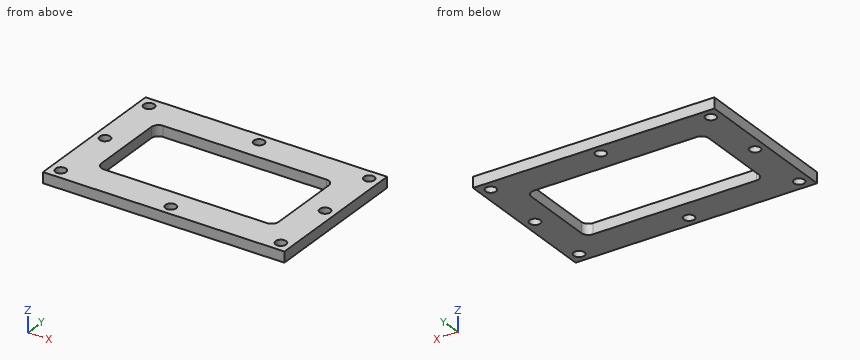
Autodesk Inventor part; units mm, degrees
ref_plane "YZ Plane" through (0, 0, 0) normal (1, 0, 0) x (0, 1, 0)
ref_plane "XZ Plane" through (0, 0, 0) normal (0, 1, 0) x (-1, 0, 0)
ref_plane "XY Plane" through (0, 0, 0) normal (0, 0, 1) x (1, 0, 0)
sketch "Sketch2" plane through (0, 0, 0) normal (0, 0, 1) x (1, 0, 0)
  line L0 (34, -21.5) -> (-34, -21.5)
  line L1 (-34, -21.5) -> (-34, 21.5)
  line L2 (-34, 21.5) -> (34, 21.5)
  line L3 (34, 21.5) -> (34, -21.5)
  line L4 (34, -21.5) -> (-34, 21.5) construction
  line L5 (-34, -21.5) -> (34, 21.5) construction
  line L6 (23, -12.5) -> (-23, -12.5)
  line L7 (-25, -10.5) -> (-25, 10.5)
  line L8 (-23, 12.5) -> (23, 12.5)
  line L9 (25, 10.5) -> (25, -10.5)
  line L10 (25, -12.5) -> (-25, 12.5) construction
  line L11 (-25, -12.5) -> (25, 12.5) construction
  arc A0 (-23, 12.5) -> (-25, 10.5) centre (-23, 10.5) ccw
  arc A1 (-25, -10.5) -> (-23, -12.5) centre (-23, -10.5) ccw
  arc A2 (23, -12.5) -> (25, -10.5) centre (23, -10.5) ccw
  arc A3 (25, 10.5) -> (23, 12.5) centre (23, 10.5) ccw
  point P0 (0, 0)
  dimension "d0" = 68
  dimension "d1" = 43
  dimension "d4" = 9
  dimension "d5" = 9
  dimension "d6" = 2
extrude "Extrusion1" add sketch "Sketch2" along normal blind 3
sketch "Sketch3" plane through (0, 0, 3) normal (0, 0, 1) x (1, 0, 0)
  line L0 (-34, -21.5) -> (34, -21.5) construction
  line L1 (34, -21.5) -> (34, 21.5) construction
  line L2 (-34, 21.5) -> (-34, -21.5) construction
  line L3 (34, 21.5) -> (-34, 21.5) construction
  line L4 (-47.6, 0) -> (47.6, 0) construction
  line L5 (0, 30.1) -> (0, -30.1) construction
  line L6 (25, 10.5) -> (25, -10.5) construction
  line L7 (-23, 12.5) -> (23, 12.5) construction
  line L8 (-25, -10.5) -> (-25, 10.5) construction
  line L9 (23, -12.5) -> (-23, -12.5) construction
  point P0 (0, 0)
  point P1 (31, -18.5)
  point P2 (31, 0)
  point P3 (31, 18.5)
  point P4 (0, 18.5)
  point P5 (-31, 18.5)
  point P6 (-31, 0)
  point P7 (-31, -18.5)
  point P8 (0, -18.5)
  dimension "d26" = 6
  dimension "d27" = 6
  dimension "d28" = 6
  dimension "d29" = 6
  dimension "d30" = 6
  dimension "d31" = 6
  dimension "d32" = 6
  dimension "d33" = 6
  dimension "d34" = 6
  dimension "d35" = 6
  dimension "d36" = 6
  dimension "d37" = 6
hole "Hole1" at (31, -18.5, 3) at (31, 0, 3) at (31, 18.5, 3) at (0, 18.5, 3) at (-31, 18.5, 3) at (-31, 0, 3) at (-31, -18.5, 3) at (0, -18.5, 3) direction (0, 0, -1) diameter 3 depth 8.8 tip angle 118
properties part number "P021_HautEcranProtecLidar"
Input: part model. Units: mm. Frame: model coordinates. Round coordinates to 2 decimals unless told otherwise and drop trailing zeros. Loops run counter-clockwise (first coordinate to the right, second up) from the corner with the lowest first, then second, coordinate; pieces in that order, holes last.
1) Material intervals for line 1 (X direction, y = -18.5, z = 2.4); line 2 (X direction, y = 0, z = 1.4); line 3 (Y direction, x = 0, z = 0.95), sorted ascending.
Ans:
line 1: x = -34 to -32.5, -29.5 to -1.5, 1.5 to 29.5, 32.5 to 34
line 2: x = -34 to -32.5, -29.5 to -25, 25 to 29.5, 32.5 to 34
line 3: y = -21.5 to -20, -17 to -12.5, 12.5 to 17, 20 to 21.5
2) Section query C-C on x = 19. Return the cut outline in (y, z).
Ans:
outline: (-21.5, 0) - (-12.5, 0) - (-12.5, 3) - (-21.5, 3) - close; (12.5, 0) - (21.5, 0) - (21.5, 3) - (12.5, 3) - close
3) Section query B-B on y = 18.5. Return the cut outline in (x, z).
Ans:
outline: (-34, 0) - (-32.5, 0) - (-32.5, 3) - (-34, 3) - close; (-29.5, 0) - (-1.5, 0) - (-1.5, 3) - (-29.5, 3) - close; (1.5, 0) - (29.5, 0) - (29.5, 3) - (1.5, 3) - close; (32.5, 0) - (34, 0) - (34, 3) - (32.5, 3) - close
4) Section query A-A on x = 31. Return the cut outline in (y, z).
Ans:
outline: (-21.5, 0) - (-20, 0) - (-20, 3) - (-21.5, 3) - close; (-17, 0) - (-1.5, 0) - (-1.5, 3) - (-17, 3) - close; (1.5, 0) - (17, 0) - (17, 3) - (1.5, 3) - close; (20, 0) - (21.5, 0) - (21.5, 3) - (20, 3) - close
5) Section query D-D on z = 0.6. Count the separate pieces of the cut face and the enclosed holes in it, plus the area to 3 significant figures.
Ans:
separate pieces: 1
enclosed holes: 9
area: 1,620 mm2
